from build123d import *

# Parameters (mm, degrees)
F0_R     = 31
F1_DEPTH = 25


# Not quite as in the source:
# - ends of sketch curves that miss each other by under 0.0002 mm in the source are joined


with BuildPart() as f1:
    # F0 (on Top) → F1 (new body)
    with BuildSketch(Plane.XY):
        with BuildLine():
            Line((-302.7446055809, 143.0378559404), (-302.7446061336, 123.0378559404))
            Line((-302.7446061336, 123.0378559404), (302.2563133603, 123.0378559404))
            Line((302.2563133603, 123.0378559404), (302.2563133603, 143.0378559404))
            ThreePointArc((302.2563133603, 143.0378559404), (281.2558506145, 164.0373893883), (302.2553878584, 185.0378521342))
            Line((302.2553878584, 185.0378521342), (302.2553878585, 205.0378483381))
            Line((302.2553878585, 205.0378483381), (-302.7446121415, 205.0378559404))
            Line((-302.7446121415, 205.0378559404), (-302.7446123928, 185.0378559404))
            ThreePointArc((-302.7446123928, 185.0378559404), (-281.7446089869, 164.0378593463), (-302.7446055809, 143.0378559404))
        make_face()
        with Locations((-216.3446089869, 164.3591374159)):
            Circle(F0_R, mode=Mode.SUBTRACT)
        with Locations((-129.9446089869, 164.3591374159)):
            Circle(F0_R, mode=Mode.SUBTRACT)
        with Locations((-43.3446089869, 164.3591374159)):
            Circle(F0_R, mode=Mode.SUBTRACT)
        with Locations((43.0553910131, 164.3591374159)):
            Circle(F0_R, mode=Mode.SUBTRACT)
        with Locations((129.4553910131, 164.3591374159)):
            Circle(F0_R, mode=Mode.SUBTRACT)
        with Locations((215.8553910131, 164.3591374159)):
            Circle(F0_R, mode=Mode.SUBTRACT)
    extrude(amount=F1_DEPTH)


solid = f1.part
Can you work these out from the model? Positions are in its coordinate system, mm. Coordinates: 2 decimals unless noted, no trailing zeros. Loops run counter-clockwise (first coordinate to the right, second up) from the corner with the lowest first, then second, coordinate; pieces in that order, holes last. Notation, with made-up numbers: (66.5, 87) - (81.5, 87) arc R26 cw to (81.5, 120) - close; hole circle Ø1 at (2.5, 55). An arc over 180 degrees is marked (long way). Answer as a JSON object with one key per item and string values. Group by question number.
Item 1: If we mould it in two halves opening along Y, with no side actions, what happens to faces 1 (the face through (4, 205.038, 12)), 2 (the face through (302.256, 133, 12)), 3 (the face through (36.335, 134.096, 12.325))? For each: released by +Y, released by -Y, zero draft, split by the parting line, or undercut.
Item 2: For pin 1 (12 mm diameter, centred on y = 160, z = 4.5, fed in from +X); pin 2 (5 mm diameter, centred on y = 156, z = 16, fed in from -X), each with a flat end and sliding along its axis, tell me the tip position at first contact or that it passes through.
Item 3: If we section it at A-A (x = 116): List the corners of the cut face in (y, z) for me.
Item 4: If we section it at D-D (x = -156): List the corners of the cut face in (y, z) for me, plus the area to 3 significant figures.
Item 5: If we section it at B-B (y = 176.5): List the corners of the cut face in (x, z) for me, plus the area to 3 significant figures.
Item 6: If we section it at C-C (z = 4.5): List the corners of the cut face in (x, y) for me, plus the area to 3 significant figures.
Item 7: If I drill on L1, parallel to Y at x = -122, z = 6.5; L2, parallel to Y at x = -26.5, z = 19.75, over which ranges is the centre line in solid material (lowest first)? Write a range as from..to.
Returned:
{
 "1": {"face 1": "released by +Y", "face 2": "zero draft", "face 3": "undercut"},
 "2": {"pin 1": "stops at x = 283.81", "pin 2": "stops at x = -284.58"},
 "3": {"outline": "(123.04, 0) - (136.43, 0) - (136.43, 25) - (123.04, 25) - close; (192.29, 0) - (205.04, 0) - (205.04, 25) - (192.29, 25) - close"},
 "4": {"outline": "(123.04, 0) - (147.56, 0) - (147.56, 25) - (123.04, 25) - close; (181.16, 0) - (205.04, 0) - (205.04, 25) - (181.16, 25) - close", "area": "1,210 mm²"},
 "5": {"outline": "(-285.84, 0) - (-244.87, 0) - (-244.87, 25) - (-285.84, 25) - close; (-187.82, 0) - (-158.47, 0) - (-158.47, 25) - (-187.82, 25) - close; (-101.42, 0) - (-71.87, 0) - (-71.87, 25) - (-101.42, 25) - close; (-14.82, 0) - (14.53, 0) - (14.53, 25) - (-14.82, 25) - close; (71.58, 0) - (100.93, 0) - (100.93, 25) - (71.58, 25) - close; (157.98, 0) - (187.33, 0) - (187.33, 25) - (157.98, 25) - close; (244.38, 0) - (285.35, 0) - (285.35, 25) - (244.38, 25) - close", "area": "5,720 mm²"},
 "6": {"outline": "(-302.74, 123.04) - (302.26, 123.04) - (302.26, 143.04) arc R21 cw to (302.26, 185.04) - (302.26, 205.04) - (-302.74, 205.04) - (-302.74, 185.04) arc R21 cw to (-302.74, 143.04) - close; hole circle Ø62 at (-216.34, 164.36); hole circle Ø62 at (-129.94, 164.36); hole circle Ø62 at (-43.34, 164.36); hole circle Ø62 at (43.06, 164.36); hole circle Ø62 at (129.46, 164.36); hole circle Ø62 at (215.86, 164.36)", "area": "30,100 mm²"},
 "7": {"L1": "y = 123.04..134.39, 194.32..205.04", "L2": "y = 123.04..138.33, 190.38..205.04"}
}
